```python
from build123d import *

# Parameters (mm, degrees)
SKETCH1_R            = 1.5
BOSS_EXTRUDE1_DEPTH  = 1.5
SKETCH2_R            = 1.5
CONNECTOR0HOLE_DEPTH = 172.17899988
CIRPATTERN1_COUNT    = 2


with BuildPart() as part:
    # Sketch1 → Boss-Extrude1 (new, symmetric)
    with BuildSketch(Plane(origin=(0, 0, 0), x_dir=(1, 0, 0), z_dir=(0, 1, 0))):
        Polygon((-10, 170), (-10, 30), (-20, 30), (-20, -30), (-10, -30), (-10, -170), (10, -170), (10, -30), (20, -30), (20, 30), (10, 30), (10, 170), align=None)
        with Locations(Location((-15.25, 15.25, 0), (0, 0, 270))):
            Circle(SKETCH1_R, mode=Mode.SUBTRACT)
        with Locations(Location((15.25, 15.25, 0), (0, 0, 270))):
            Circle(SKETCH1_R, mode=Mode.SUBTRACT)
        with Locations(Location((15.25, -15.25, 0), (0, 0, 270))):
            Circle(SKETCH1_R, mode=Mode.SUBTRACT)
        with Locations(Location((-15.25, -15.25, 0), (0, 0, 270))):
            Circle(SKETCH1_R, mode=Mode.SUBTRACT)
    extrude(amount=BOSS_EXTRUDE1_DEPTH, both=True)

    # Sketch2 → connector0hole (cut, symmetric)
    with BuildSketch(Plane(origin=(0, 0, 0), x_dir=(1, 0, 0), z_dir=(0, 1, 0))):
        with Locations(Location((-6, 165, 0), (0, 0, 270))):
            Circle(SKETCH2_R)
        with Locations(Location((6, 165, 0), (0, 0, 270))):
            Circle(SKETCH2_R)
    connector0hole = extrude(amount=CONNECTOR0HOLE_DEPTH, both=True, mode=Mode.SUBTRACT)

    # CirPattern1: connector0hole ×2 about axis
    cirpattern1_axis = Axis((0, 0, 0), (0, 1, 0))
    for i in range(1, CIRPATTERN1_COUNT):
        add(connector0hole.rotate(cirpattern1_axis, i * 360 / CIRPATTERN1_COUNT), mode=Mode.SUBTRACT)


solid = part.part
```
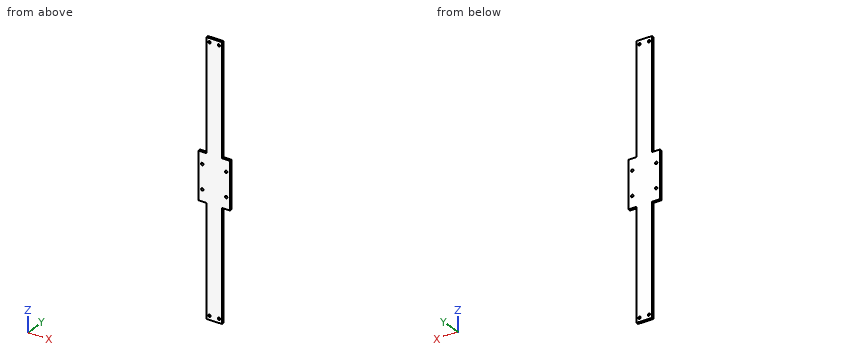
Can you work these out from the model? Positions are in its coordinate system, mm. Give positions to 0.01 mm unless a question says otherwise; leave off trailing zeros. Order: outer loops, then holes, each group sorted by start corner. A loop starts at its lowest first (then second) coordinate and runs counter-clockwise, first axis right, second up. Notation, with made-up numbers: (43.25, 18) - (66.25, 18) arc R21 ccw to (66.25, 38) - close; hole circle Ø6 at (-30.5, 56). An arc over 180 degrees is marked (long way). Use a Markdown table: item, result. Add a question column.
Q1. If we section it at A-A on y = 0.25: Count the separate pieces of the cut face and the enclosed holes in it, plus the area to 3 significant figures.
Q2. Please list where these lines run through material, in increasing order: line 1 along X through (y, z) = (-0.05, 15.25); line 2 along Z through (x, y) = (-6, -0.5); line 3 along X through (y, z) = (-0.2, -165).
Q3. I'm going to push flat-ended pins straight in: pin 1 (1.5 mm diameter, centred on y = -0.5, z = -114, fed in from -X); pin 2 (0.9 mm diameter, centred on y = 0, z = -103.5, fed in from +X); pin 3 (1.5 mm diameter, centred on x = 14, y = 0, fed in from +Z). Where does each tip first touch, or does it pass through?
Q4. If we section it at B-B on z = 106: Write out the boundary of the cut face in (x, y), plus the area to 3 significant figures.
Answers follow:
| question | item | result |
|---|---|---|
| 1 | separate pieces | 1 |
| 1 | enclosed holes | 8 |
| 1 | area | 7,940 mm^2 |
| 2 | line 1 | x = -20 to -16.75, -13.75 to 13.75, 16.75 to 20 |
| 2 | line 2 | z = -170 to -166.5, -163.5 to 163.5, 166.5 to 170 |
| 2 | line 3 | x = -10 to -7.5, -4.5 to 4.5, 7.5 to 10 |
| 3 | pin 1 | stops at x = -10 |
| 3 | pin 2 | stops at x = 10 |
| 3 | pin 3 | stops at z = 30 |
| 4 | outline | (-10, -1.5) - (10, -1.5) - (10, 1.5) - (-10, 1.5) - close |
| 4 | area | 60.0 mm^2 |
